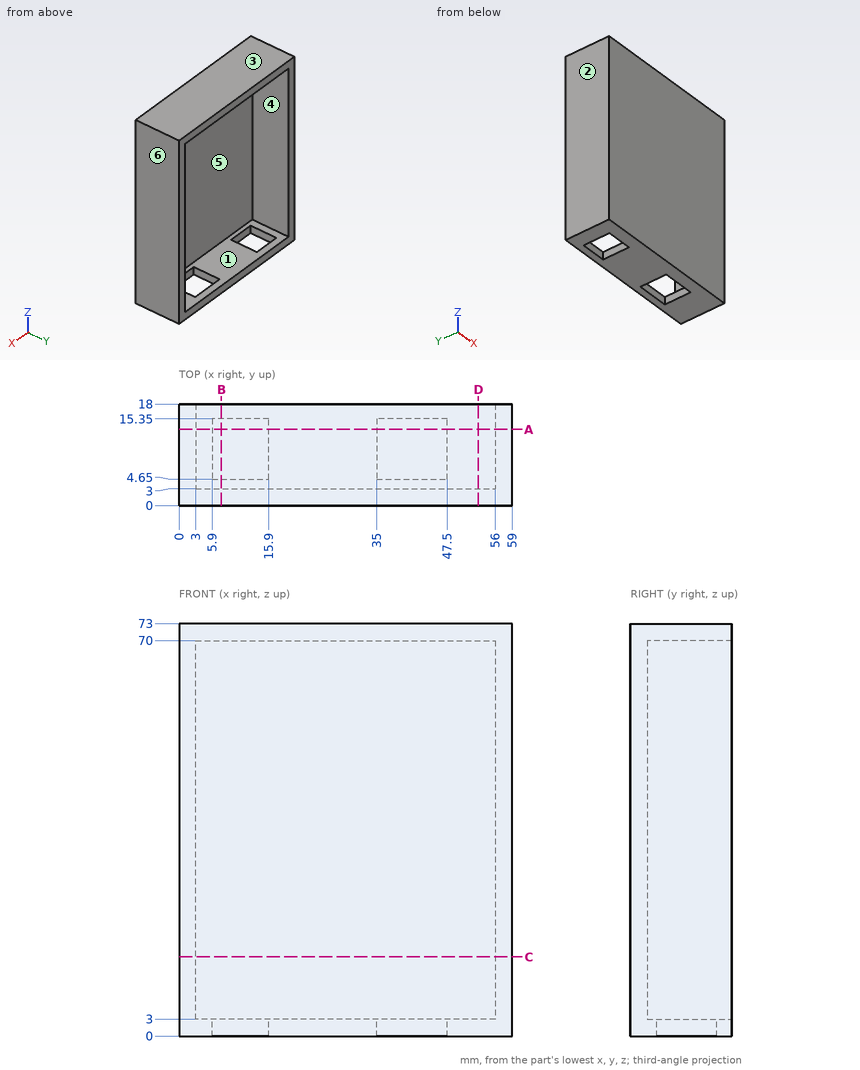
Geometry check sheet. Reference: drawing and pictorial views, mm from the part's lowest x, y, z. A direction names the side the tool comes from. Round coordinates to 2 decimals unless told otherwise and drop trailing zeros. Order: outer loops, then holes, each group sorted by start corner. A loop starts at its lowest first (then second) coordinate and runs counter-clockwise, first axis right, second up. Notation, with made-up numbers: M 29.5,-5 L 74.5,-5 A27 cw 74.5,19 Z; hole C 71.5,67 d1. An arc over 180 degrees is marked long. Write item = value, one per line.
Q1. Section check C-C (z = 14). Enter the section's corners in (x, y), plus the area to 3 significant figures.
Answer block:
outline = M 0,0 L 59,0 L 59,18 L 56,18 L 56,3 L 3,3 L 3,18 L 0,18 Z
area = 267 mm^2
Q2. Section check A-A (y = 13.5). Enter the section's corners in (x, z).
Answer block:
outline = M 0,0 L 5.9,0 L 5.9,3 L 3,3 L 3,70 L 56,70 L 56,3 L 47.5,3 L 47.5,0 L 59,0 L 59,73 L 0,73 Z; M 15.9,0 L 35,0 L 35,3 L 15.9,3 Z
Q3. Section check B-B (x = 7.5). Enter the section's corners in (y, z).
Answer block:
outline = M 0,0 L 4.65,0 L 4.65,3 L 3,3 L 3,70 L 18,70 L 18,73 L 0,73 Z; M 15.35,0 L 18,0 L 18,3 L 15.35,3 Z
Q4. Release check for a two-part mould opening along Z. For the marked faces 3, 4, 5 and 6 record: released by +Z, released by -Z, zero draft, split by the parting line, or undercut.
Answer block:
face_3 = released by +Z
face_4 = undercut
face_5 = undercut
face_6 = zero draft
Q5. Scan lines: line 1 (X direction, y = 6.5, z = 16); line 2 (Z direction, x = 24, y = 3.25); line 3 (Z direction, x = 38.5, y = 12.75). Record each from-to range of solid material in increasing order.
Answer block:
line_1 = 0 to 3, 56 to 59
line_2 = 0 to 3, 70 to 73
line_3 = 70 to 73
Q6. Set-up check for the marked faces 1 and 2: record each of +Z, -Z, +X, -X, +Y, -Y from which the full face is reachable in a straight line by a thin tool's end or side.
Answer block:
face_1 = +Y
face_2 = +Z, -Z, -X, +Y, -Y
Q7. Section check D-D (x = 53). Enter the section's corners in (y, z).
Answer block:
outline = M 0,0 L 18,0 L 18,3 L 3,3 L 3,70 L 18,70 L 18,73 L 0,73 Z
Q8. Depth check by flat-ended pin: pin 1 Ø12 at (x, z) = (40, 31.5) entering from +Y. Enter the tip coordinate at first touch or a pass-through.
Answer block:
pin_1 = 3
